```python
from build123d import *

# Parameters (mm, degrees)
SKETCH_1_W                  = 86
SKETCH_1_H                  = 44.2
EXTRUDE_1_DEPTH             = 14.2
EXTRUDE_2_DEPTH             = 5
SKETCH_3_W                  = 19.825
SKETCH_3_H                  = 42.4
CUT_EXTRUDE_1_DEPTH         = 18.3
SKETCH_4_W                  = 19.375
SKETCH_4_H                  = 42.4
CUT_EXTRUDE_2_DEPTH         = 18.3
SKETCH_5_W                  = 19.375
SKETCH_5_H                  = 42.4
CUT_EXTRUDE_3_DEPTH         = 18.3
SKETCH_6_W                  = 19.825
SKETCH_6_H                  = 42.4
CUT_EXTRUDE_4_DEPTH         = 18.3
HOLE_WIZARD_8_3_8_3_1_D     = 8.3
HOLE_WIZARD_8_3_8_3_1_DEPTH = 3.2
HOLE_WIZARD_5_0_5_1_D       = 5
HOLE_WIZARD_5_0_5_1_DEPTH   = 0.9
HOLE_WIZARD_5_0_5_2_D       = 5
HOLE_WIZARD_5_0_5_2_DEPTH   = 0.9
HOLE_WIZARD_5_0_5_3_D       = 5
HOLE_WIZARD_5_0_5_3_DEPTH   = 0.9
FILLET_1_R                  = 3
EXTRUDE_START               = -3.5
SKETCH_15_R                 = 4.15
EXTRUDE_3_DEPTH             = 3.5
FILLET_3_R                  = 2


with BuildPart() as part:
    # Эскиз1 → Бобышка-Вытянуть1 (new body)
    with BuildSketch(Plane.XY.offset(9.6)):
        with Locations((47, 0)):
            Rectangle(SKETCH_1_W, SKETCH_1_H)
    extrude(amount=-EXTRUDE_1_DEPTH)

    # Эскиз2 → Бобышка-Вытянуть2 (add)
    with BuildSketch(Plane(origin=(0, 0, -4.6), x_dir=(-1, 0, 0), z_dir=(0, 0, -1))):
        with BuildLine():
            Line((-90, -22.1), (-90, -17.1))
            ThreePointArc((-90, -17.1), (-104, 0), (-90, 17.1))
            Line((-90, 17.1), (-90, 22.1))
            Line((-90, 22.1), (-4, 22.1))
            Line((-4, 22.1), (-4, -22.1))
            Line((-4, -22.1), (-90, -22.1))
        make_face()
        with BuildLine():
            Line((-90, -12.994779171), (-90, 12.994779171))
            ThreePointArc((-90, 12.994779171), (-100, 0), (-90, -12.994779171))
        make_face(mode=Mode.SUBTRACT)
    extrude(amount=EXTRUDE_2_DEPTH)

    # Эскиз3 → Вырез-Вытянуть1 (cut)
    with BuildSketch(Plane.XY.offset(9.6)):
        with Locations((79.1875, 0)):
            Rectangle(SKETCH_3_W, SKETCH_3_H)
    extrude(amount=-CUT_EXTRUDE_1_DEPTH, mode=Mode.SUBTRACT)

    # Эскиз4 → Вырез-Вытянуть2 (cut)
    with BuildSketch(Plane.XY.offset(9.6)):
        with Locations((58.6875, 0)):
            Rectangle(SKETCH_4_W, SKETCH_4_H)
    extrude(amount=-CUT_EXTRUDE_2_DEPTH, mode=Mode.SUBTRACT)

    # Эскиз5 → Вырез-Вытянуть3 (cut)
    with BuildSketch(Plane.XY.offset(9.6)):
        with Locations((38.4125, 0)):
            Rectangle(SKETCH_5_W, SKETCH_5_H)
    extrude(amount=-CUT_EXTRUDE_3_DEPTH, mode=Mode.SUBTRACT)

    # Эскиз6 → Вырез-Вытянуть4 (cut)
    with BuildSketch(Plane.XY.offset(9.6)):
        with Locations((17.9125, 0)):
            Rectangle(SKETCH_6_W, SKETCH_6_H)
    extrude(amount=-CUT_EXTRUDE_4_DEPTH, mode=Mode.SUBTRACT)

    # Диаметр отверстия Ø8.3 (8.3)1
    with Locations(Plane.ZY.offset(-4)):
        with Locations((0, 0)):
            Hole(HOLE_WIZARD_8_3_8_3_1_D / 2, depth=HOLE_WIZARD_8_3_8_3_1_DEPTH)

    # Диаметр отверстия Ø5.0 (5)1
    with Locations(Plane(origin=(28.725, 0, 0), x_dir=(0, 0, -1), z_dir=(1, 0, 0))):
        with Locations((-9.6, 0)):
            Hole(HOLE_WIZARD_5_0_5_1_D / 2, depth=HOLE_WIZARD_5_0_5_1_DEPTH)

    # Диаметр отверстия Ø5.0 (5)2
    with Locations(Plane.ZY.offset(-48.1)):
        with Locations((9.6, 0)):
            Hole(HOLE_WIZARD_5_0_5_2_D / 2, depth=HOLE_WIZARD_5_0_5_2_DEPTH)

    # Диаметр отверстия Ø5.0 (5)3
    with Locations(Plane.ZY.offset(-68.375)):
        with Locations((9.6, 0)):
            Hole(HOLE_WIZARD_5_0_5_3_D / 2, depth=HOLE_WIZARD_5_0_5_3_DEPTH)

    # Скругление1
    fillet_1_edges = [part.edges().sort_by_distance(p)[0] for p in [
        (4, -22.1, 0),
        (4, 22.1, 0),
    ]]
    fillet(fillet_1_edges, radius=FILLET_1_R)

    # Эскиз15 → Бобышка-Вытянуть3 (add)
    with BuildSketch(Plane.ZY.offset(-4).offset(EXTRUDE_START)):
        Circle(SKETCH_15_R)
    extrude(amount=EXTRUDE_3_DEPTH)

    # Скругление3
    fillet_3_edges = [part.edges().sort_by_distance(p)[0] for p in [
        (90, -15.047389586, -4.6),
        (90, 15.047389586, -4.6),
        (79.1875, 21.2, -8.7),
        (69.275, 21.2, 0.45),
        (89.1, 0, -8.7),
        (89.1, 21.2, 0.45),
        (79.1875, -21.2, -8.7),
        (89.1, -21.2, 0.45),
        (69.275, 0, -8.7),
        (69.275, -21.2, 0.45),
        (49, 0, -8.7),
        (49, -21.2, 0.45),
        (58.6875, 21.2, -8.7),
        (49, 21.2, 0.45),
        (68.375, 0, -8.7),
        (68.375, 21.2, 0.45),
        (58.6875, -21.2, -8.7),
        (68.375, -21.2, 0.45),
        (28.725, 0, -8.7),
        (28.725, -21.2, 0.45),
        (38.4125, 21.2, -8.7),
        (28.725, 21.2, 0.45),
        (48.1, 0, -8.7),
        (48.1, 21.2, 0.45),
        (38.4125, -21.2, -8.7),
        (48.1, -21.2, 0.45),
        (17.9125, -21.2, -8.7),
        (27.825, -21.2, 0.45),
        (8, 0, -8.7),
        (8, -21.2, 0.45),
        (17.9125, 21.2, -8.7),
        (8, 21.2, 0.45),
        (27.825, 0, -8.7),
        (27.825, 21.2, 0.45),
    ]]
    fillet(fillet_3_edges, radius=FILLET_3_R)


solid = part.part
```
Design review of the part built by this model. Coordinates are the model's own, in mm. Give positions to 0.01 mm unless a question says otherwise; leave off trailing zeros. Order: outer loops, then holes, each group sorted by start corner. A loop starts at its lowest first (then second) coordinate and runs counter-clockwise, first axis right, second up. Notation, with made-up numbers: M 22.5,63 L 46.5,63 A19 cw 46.5,94 Z; hole C 71.5,33 d1. An arc over 180 degrees is marked long. One line per question, with ' | ' between items. Start each with the question number.
Q1. The part is to be moulded in two halves that separate along Y. For faces 1 (the face through (79, 21.2, 2)), 2 (the face through (68.375, 0, 2)), 3 (the face through (104, 0, -7)), 4 (the face through (90.57, 14.73, -4)), say which applies: +Y half, -Y half, draft (parallel to the pull), parting line (faces both ways), or undercut.
Q2. We need section D-D (z = 2). State how many separate pieces and enclosed holes the cut face has, plus the area to 3 significant figures.
Q3. For L1, parallel to X at y = -16.5, z = -2.25 (3 decimals); L2, parallel to Y at x = 23.5, z = -3.75; L3, parallel to X at y = 20.5, z = 7, list the stretches that pass through material, from the lowest coordinate up. Write a range as [from, to].
Q4. For pin 1 Ø4.5 at (x, y) = (40.5, -4) entering from +Z; pin 2 Ø8 at (y, z) = (4, -0.5) entering from +X; pin 3 Ø8 at (y, z) = (2.5, -2.5) entering from +X, all flat-tipped, find the tip position at first contact; note any pin that passes through.
Q5. We need section B-B (x = 60.5). Write out the cut boundary in (y, z).
Returned:
1) face 1: undercut | face 2: undercut | face 3: parting line | face 4: draft
2) separate pieces: 1 | enclosed holes: 4 | area: 487 mm2
3) L1: [4, 8], [27.825, 28.725], [48.1, 49], [68.375, 69.275], [89.1, 90] | L2: [-22.1, -21.2], [21.2, 22.1] | L3: [4.35, 8.48], [27.34, 29.21], [47.62, 49.48], [67.89, 69.76], [88.62, 90]
4) pin 1: z = -8.7 | pin 2: x = 90 | pin 3: x = 104
5) outline: M -22.1,-9.6 L 22.1,-9.6 L 22.1,9.6 L 21.2,9.6 L 21.2,-6.7 A2 cw 19.2,-8.7 L -19.2,-8.7 A2 cw -21.2,-6.7 L -21.2,9.6 L -22.1,9.6 Z
